```python
from build123d import *

# Parameters (mm, degrees)
BOSS_EXTRUDE1_DEPTH = 197.612


with BuildPart() as part:
    # Sketch1 → Boss-Extrude1 (new body)
    with BuildSketch(Plane(origin=(0, 0, -228.6), x_dir=(-1, 0, 0), z_dir=(0, 0, -1))):
        with BuildLine():
            Line((3.805488829, -6.0833), (7.171036753, -0.254))
            ThreePointArc((7.171036753, -0.254), (7.239095848, 0), (7.171036753, 0.254))
            Line((7.171036753, 0.254), (3.805488829, 6.0833))
            ThreePointArc((3.805488829, 6.0833), (3.619547924, 6.269240905), (3.365547924, 6.3373))
            Line((3.365547924, 6.3373), (-3.365547924, 6.3373))
            ThreePointArc((-3.365547924, 6.3373), (-3.619547924, 6.269240905), (-3.805488829, 6.0833))
            Line((-3.805488829, 6.0833), (-7.171036753, 0.254))
            ThreePointArc((-7.171036753, 0.254), (-7.239095848, 0), (-7.171036753, -0.254))
            Line((-7.171036753, -0.254), (-3.805488829, -6.0833))
            ThreePointArc((-3.805488829, -6.0833), (-3.619547924, -6.269240905), (-3.365547924, -6.3373))
            Line((-3.365547924, -6.3373), (3.365547924, -6.3373))
            ThreePointArc((3.365547924, -6.3373), (3.619547924, -6.269240905), (3.805488829, -6.0833))
        make_face()
    extrude(amount=-BOSS_EXTRUDE1_DEPTH)


solid = part.part
```
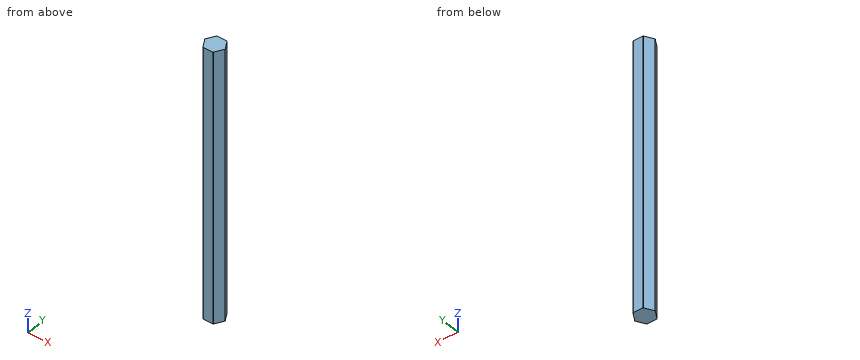
Build history of the part. All positions in model axes, mm. Round coordinates to 2 decimals unless told otherwise and drop trailing zeros. Write each loop counter-clockwise with the first axis right and the second up, starting at its lowest first coordinate (ties: lowest second). Pieces come first, ordered by that corner, then holes.
1) Band-saw the part on B-B, the plane y = -4.25. List the corners of the cut face in (x, z).
2) Pin check, flat tips, straight feed: pin 1 (2 mm diameter, centred on y = 5, z = -196, fed in from +X); pin 2 (1.5 mm diameter, centred on y = -3.5, z = -178, fed in from +X); pin 3 (5 mm diameter, centred on y = -3.5, z = -102, fed in from +X). Stop position of each tip, or through.
3) Drill centre lines: probe 1 along Y at (x, z) = (4, -195.5); probe 2 along X at (y, z) = (2.25, -152); probe 3 along X at (y, z) = (-5.25, -48). Where is each one in solid material? Low to high.
4) Band-saw the part on C-C, the plane x = -5.5. List the corners of the cut face in (y, z).
5) Band-saw the part on A-A, the plane z = -128. List the corners of the cut face in (x, y), and give its area (3 significant figures).
Ans:
1. outline: (-4.86, -228.6) - (4.86, -228.6) - (4.86, -30.99) - (-4.86, -30.99) - close
2. pin 1: stops at x = 5.01
2. pin 2: stops at x = 5.73
2. pin 3: stops at x = 6.74
3. probe 1: y = -5.75 to 5.75
3. probe 2: x = -6.02 to 6.02
3. probe 3: x = -4.29 to 4.29
4. outline: (-3.15, -228.6) - (3.15, -228.6) - (3.15, -30.99) - (-3.15, -30.99) - close
5. outline: (-7.17, -0.25) - (-3.81, -6.08) arc R0.51 ccw to (-3.37, -6.34) - (3.37, -6.34) arc R0.51 ccw to (3.81, -6.08) - (7.17, -0.25) arc R0.51 ccw to (7.17, 0.25) - (3.81, 6.08) arc R0.51 ccw to (3.37, 6.34) - (-3.37, 6.34) arc R0.51 ccw to (-3.81, 6.08) - (-7.17, 0.25) arc R0.51 ccw to start
5. area: 139 mm2
